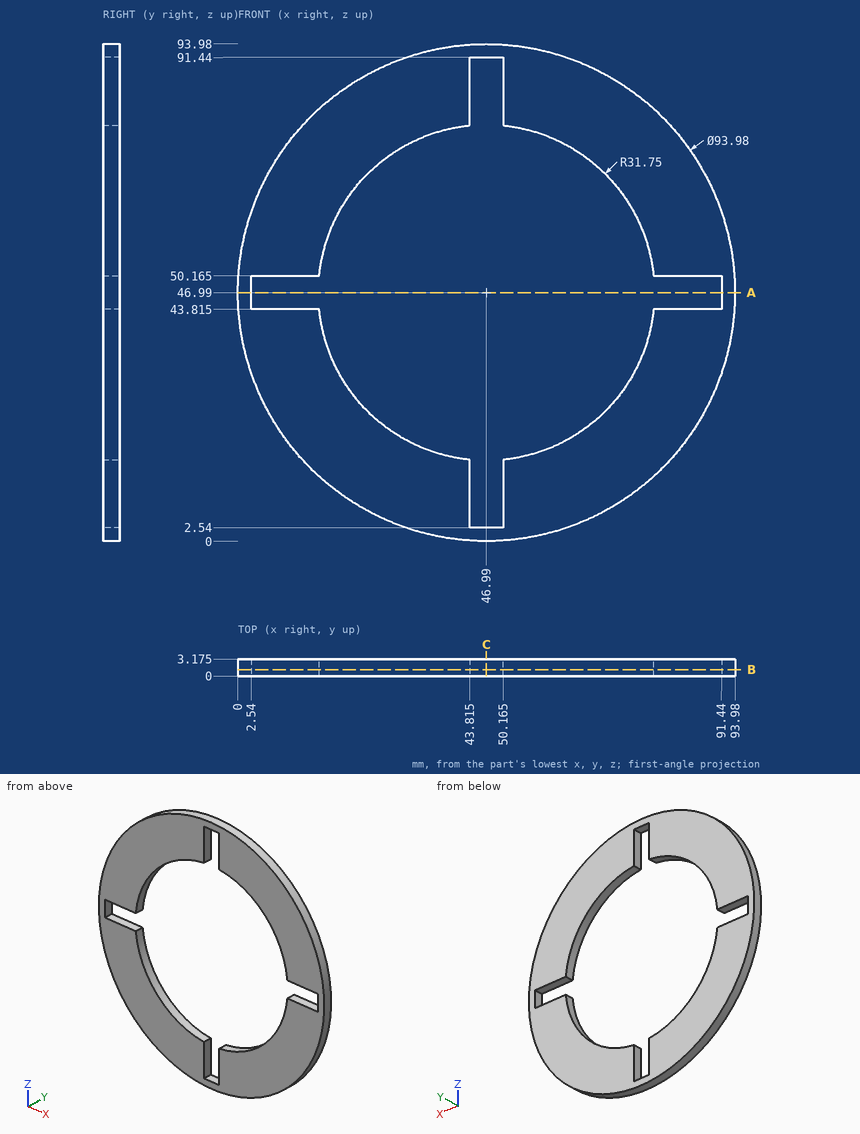
Here's the drawing with two shaded views (mm, measured from the low corner). I have some questions. Round coordinates to 2 decimals unless told otherwise and drop trailing zeros. Loops run counter-clockwise (first coordinate to the right, second up) from the corner with the lowest first, then second, coordinate; pieces in that order, holes last. Notation, with made-up numbers: M -34.75,34 L -23.75,34 A27 cw -23.75,65 Z; hole C 29.5,-38 d5. An arc over 180 degrees is marked long. Answer as a JSON object with one key per item and string values. Group by question number.
Q1. Imagine slicing it at C-C, the plane x = 46.99. Please give me the cut outline in (y, z) (3 decimals).
Q2. Imagine slicing it at B-B, the plane y = 1.2. Please give me the cut outline in (x, z) (3 decimals), then the cut area to 3 significant figures.
Q3. Please list where these lines run through material, in increasing order: L1, parallel to Z at x = 63, y = 1.1; L2, parallel to Z at x = 10.5, y = 1.6 (3 decimals); L3, parallel to X at y = 1.9, z = 71.5.
Q4. Will these pins go through, and if not, where does the flat tip stop? pin 1 (1 mm diameter, centred on x = 15, y = 2.5, fed in from +Z); pin 2 (1.6 mm diameter, centred on x = 10, y = 2, fed in from +Z); pin 3 (1 mm diameter, centred on y = 2, z = 47.5, fed in from +X).
Q5. Imagine slicing it at A-A, the plane z = 46.99. Please give me the cut outline in (x, y) (3 decimals).
Findings:
{
 "1": {"outline": "M 0,0 L 3.175,0 L 3.175,2.54 L 0,2.54 Z; M 0,91.44 L 3.175,91.44 L 3.175,93.98 L 0,93.98 Z"},
 "2": {"outline": "C 46.99,46.99 d93.98; hole M 2.54,43.815 L 15.399,43.815 A31.75 ccw 43.815,15.399 L 43.815,2.54 L 50.165,2.54 L 50.165,15.399 A31.75 ccw 78.581,43.815 L 91.44,43.815 L 91.44,50.165 L 78.581,50.165 A31.75 ccw 50.165,78.581 L 50.165,91.44 L 43.815,91.44 L 43.815,78.581 A31.75 ccw 15.399,50.165 L 2.54,50.165 Z", "area": "3,450 mm2"},
 "3": {"L1": "z = 2.81 to 19.57, 74.41 to 91.17", "L2": "z = 17.384 to 43.815, 50.165 to 76.596", "L3": "x = 6.9 to 26.81, 67.17 to 87.08"},
 "4": {"pin 1": "stops at z = 81.87", "pin 2": "stops at z = 76.96", "pin 3": "stops at x = 93.98"},
 "5": {"outline": "M 0,0 L 2.54,0 L 2.54,3.175 L 0,3.175 Z; M 91.44,0 L 93.98,0 L 93.98,3.175 L 91.44,3.175 Z"}
}
